CAD build for the part. Positions are in the model's coordinates, mm. A direction names the side the tool comes from. Give positions to 0.01 mm unless a question says otherwise; leave off trailing zeros. Write each loop counter-clockwise with the first axis right and the second up, starting at its lowest first coordinate (ties: lowest second). Pieces come first, ordered by that corner, then holes. Notation, with made-up numbers: (14, 72.5) - (72, 72.5) arc R18 ccw to (72, 91.5) - close; hole circle Ø6 at (80, 12.5). An arc over 180 degrees is marked (long way). Answer as a JSON object with one key per item and string values.
from build123d import *

# Parameters (mm, degrees)
SKETCH1_W           = 40
SKETCH1_H           = 40.4
BOSS_EXTRUDE1_DEPTH = 20
SKETCH3_W           = 3
SKETCH3_H           = 20
BOSS_EXTRUDE2_DEPTH = 7.25
SKETCH5_R           = 1.938887877
SKETCH5_R_2         = 1.98650292
CUT_EXTRUDE1_DEPTH  = 7.25
SKETCH6_R           = 7.5
BOSS_EXTRUDE3_DEPTH = 10
BOSS_EXTRUDE4_DEPTH = 5


with BuildPart() as part:
    # Sketch1 → Boss-Extrude1 (new body)
    with BuildSketch(Plane(origin=(0, 0, 0), x_dir=(1, 0, 0), z_dir=(0, 1, 0))):
        with Locations((-7.684478372, -4.939949109)):
            Rectangle(SKETCH1_W, SKETCH1_H)
    extrude(amount=BOSS_EXTRUDE1_DEPTH)

    # Sketch3 → Boss-Extrude2 (add)
    with BuildSketch(Plane(origin=(12.315521628, 0, 0), x_dir=(0, 0, -1), z_dir=(1, 0, 0))):
        with Locations((-13.939949109, 10)):
            Rectangle(SKETCH3_W, SKETCH3_H)
    boss_extrude2 = extrude(amount=BOSS_EXTRUDE2_DEPTH)

    # Mirror1: Boss-Extrude2 across plane
    add(boss_extrude2.mirror(Plane.ZY.offset(7.684478372)))

    # Sketch5 → Cut-Extrude1 (cut)
    with BuildSketch(Plane.XY.offset(15.439949109)):
        with Locations((15.940521628, 15)):
            Circle(SKETCH5_R)
        with Locations((15.940521628, 5)):
            Circle(SKETCH5_R_2)
    cut_extrude1 = extrude(amount=-CUT_EXTRUDE1_DEPTH, mode=Mode.SUBTRACT)

    # Mirror2: Cut-Extrude1 across plane
    add(cut_extrude1.mirror(Plane.ZY.offset(7.684478372)), mode=Mode.SUBTRACT)

    # Sketch6 → Boss-Extrude3 (add)
    with BuildSketch(Plane.XY.offset(25.139949109)):
        with Locations((2.315521628, 10)):
            Circle(SKETCH6_R)
    extrude(amount=BOSS_EXTRUDE3_DEPTH)

    # Sketch8 → Boss-Extrude4 (add)
    with BuildSketch(Plane.XY.offset(35.139949109)):
        with BuildLine():
            Line((10.818468117, 7.39802315), (23.828352366, 7.39802315))
            ThreePointArc((23.828352366, 7.39802315), (25.779835003, 9.349505788), (23.828352366, 11.300988425))
            Line((23.828352366, 11.300988425), (10.818468117, 11.300988425))
            ThreePointArc((10.818468117, 11.300988425), (9.571889646, 11.847462314), (9.129094063, 13.1345224))
            ThreePointArc((9.129094063, 13.1345224), (-5.184055447, 10.07964725), (9.060986037, 6.72147748))
            ThreePointArc((9.060986037, 6.72147748), (9.876866117, 7.223046033), (10.818468117, 7.39802315))
        make_face()
    extrude(amount=-BOSS_EXTRUDE4_DEPTH)


solid = part.part
(1) Saw through at B-B, the plane x = 4. Give the cut face in (y, z), and give its area (3 significant figures).
Answer key:
{"outline": "(0, -15.26) - (20, -15.26) - (20, 25.14) - (17.31, 25.14) - (17.31, 35.14) - (2.69, 35.14) - (2.69, 25.14) - (0, 25.14) - close", "area": "954 mm²"}
(2) Saw through at A-A, the plane y = 5. Give the cut face in (x, z), and give its area (3 significant figures).
Answer key:
{"outline": "(-34.93, 12.44) - (-33.3, 12.44) - (-33.3, 15.44) - (-34.93, 15.44) - close; (-29.32, 12.44) - (-27.68, 12.44) - (-27.68, -15.26) - (12.32, -15.26) - (12.32, 12.44) - (13.95, 12.44) - (13.95, 15.44) - (12.32, 15.44) - (12.32, 25.14) - (7.91, 25.14) - (7.91, 35.14) - (-3.27, 35.14) - (-3.27, 25.14) - (-27.68, 25.14) - (-27.68, 15.44) - (-29.32, 15.44) - close; (17.93, 12.44) - (19.57, 12.44) - (19.57, 15.44) - (17.93, 15.44) - close", "area": "1,750 mm²"}
(3) Flat gauge pins, fed straight in: P1, Ø5, axis at y = 9, z = 19.5, coming from the +X side; P2, Ø3, axis at y = 6, z = 19, coming from the -X side; P3, Ø3, axis at x = -31.31, y = 5, coming from the -Z side; P4, Ø3, axis at y = 2, z = 15, coming from the +X side. Where does each tip first touch, or does it go through?
Answer key:
{"P1": "stops at x = 12.32", "P2": "stops at x = -27.68", "P3": "passes through", "P4": "stops at x = 19.57"}
(4) 3-axis set-ups, long thin cutter, end or side, ignore diameter. For faces 4 (the face through (9.864, 7.218, 32.675)), 5 (the face through (17, 11.301, 33)), 6 (the face through (-31, 10, 15.44)): which of +Z, -Z, +X, -X, +Y, -Y reach the whole face in a straight line?
Answer key:
{"face 4": "+Z, +X, -Y", "face 5": "+Z, +X, +Y", "face 6": "+Z, -X, +Y, -Y"}
(5) Probe L1, parallel to Z at x = -22, y = 3; L2, parallel to Z at x = -28, y = 10; L3, parallel to X at y = 8.75, z = 17.5. List the from-to ranges inside material, lowest first. Write a range as [from, to].
Answer key:
{"L1": "z = [-15.26, 25.14]", "L2": "z = [12.44, 15.44]", "L3": "x = [-27.68, 12.32]"}
(6) Saw through at C-C, the plane z = 18. Give the cut face in (x, y).
Answer key:
{"outline": "(-27.68, 0) - (12.32, 0) - (12.32, 20) - (-27.68, 20) - close"}
(7) Pull direction X, two halves, no side cores. Call faces 1 (the face through (-31, 10, 12.44)), 2 (the face through (19.566, 10, 14)), 3 (the face through (14.476, 6.343, 13.961)): pulls with the +X half, pulls with the -X half, needs draft (parallel to the pull), parting line crosses it, or undercut.
Answer key:
{"face 1": "needs draft", "face 2": "pulls with the +X half", "face 3": "undercut"}
(8) Saw through at D-D, the plane y = 10. Give the cut face in (x, z), and give its area (3 significant figures).
Answer key:
{"outline": "(-34.93, 12.44) - (-27.68, 12.44) - (-27.68, -15.26) - (12.32, -15.26) - (12.32, 12.44) - (19.57, 12.44) - (19.57, 15.44) - (12.32, 15.44) - (12.32, 25.14) - (9.82, 25.14) - (9.82, 30.14) - (25.67, 30.14) - (25.67, 35.14) - (-5.18, 35.14) - (-5.18, 25.14) - (-27.68, 25.14) - (-27.68, 15.44) - (-34.93, 15.44) - close", "area": "1,890 mm²"}
